The model under review builds one solid part; all positions refer to its coordinate system, in mm. Face numbers are marked on the shaded views. A direction names the side the tool comes from. Coordinates: 2 decimals unless noted, no trailing zeros. Loops run counter-clockwise (first coordinate to the right, second up) from the corner with the lowest first, then second, coordinate; pieces in that order, holes last. Notation, with made-up numbers: (-0.75, 53) - (33.25, 53) arc R29 ccw to (33.25, 73) - close; hole circle Ø11 at (3, 42.25). An arc over 180 degrees is marked (long way). One line per item, written item: value. Start each with the question number.
1. We need section B-B, the plane y = 53.5. Give the boundary of the cut face in (x, z), then the cut area to 3 significant figures.
2. Insertion check: P1, Ø10, axis at x = 12.5, z = 32, coming from the -Y side; P2, Ø12, axis at y = 43.5, z = 45.5, coming from the +X side; P3, Ø8, axis at x = -28.5, z = 54, coming from the +Y side; P4, Ø1, axis at x = 20.5, y = 46.5, coming from the -Z side. Each pin has a flat end and moves straight along its axis. Give the tip position at first contact, or say it passes through.
3. We need section C-C, the plane x = -35.5. Give the boundary of the cut face in (y, z), then the cut area to 3 significant figures.
4. For the marked faces 1 and 2, list the 3-axis set-ups (+Z, -Z, +X, -X, +Y, -Y) from which the entire face can be reached by the end or side of a thin tool; tool diameter is ignored.
5. We need section D-D, the plane x = 0. Give the boundary of the cut face in (y, z), then the cut area to 3 significant figures.
6. To check wall thickness, follow line 1 (X direction, y = 53.75, z = 0); line 2 (Y direction, x = 17, z = 51.5); line 3 (Z direction, x = 9.5, y = 48). State the ranges of each line that lie inside material, in increasing order.
7. We need section A-A, the plane z = 0. Give the boundary of the cut face in (x, y), then the cut area to 3 significant figures.
from build123d import *

# Parameters (mm, degrees)
SKETCH1_R           = 72
BOSS_EXTRUDE4_DEPTH = 50
SKETCH5_R           = 72
SKETCH5_R_2         = 69
BOSS_EXTRUDE5_DEPTH = 7


with BuildPart() as part:
    # Sketch1 → Boss-Extrude4 (new body)
    with BuildSketch(Plane(origin=(0, 0, 0), x_dir=(1, 0, 0), z_dir=(0, 1, 0))):
        with Locations(Location((0, 0, 0), (0, 0, 270))):
            Circle(SKETCH1_R)
    extrude(amount=BOSS_EXTRUDE4_DEPTH)

    # Sketch4 → Cut-Revolve2 (revolve, cut)
    with BuildSketch(Plane.XY, mode=Mode.PRIVATE) as cut_revolve2_sk:
        with BuildLine():
            Line((0, 50), (42, 50))
            ThreePointArc((42, 50), (29.69848481, 20.30151519), (0, 8))
            Line((0, 8), (0, 50))
        make_face()
    revolve(cut_revolve2_sk.sketch.rotate(Axis((0, 50, 0), (0, -1, 0)), 180), axis=Axis((0, 50, 0), (0, -1, 0)), mode=Mode.SUBTRACT)

    # Sketch5 → Boss-Extrude5 (add)
    with BuildSketch(Plane(origin=(0, 50, 0), x_dir=(1, 0, 0), z_dir=(0, 1, 0))):
        with Locations(Location((0, 0, 0), (0, 0, 270))):
            Circle(SKETCH5_R)
        with Locations(Location((0, 0, 0), (0, 0, 270))):
            Circle(SKETCH5_R_2, mode=Mode.SUBTRACT)
    extrude(amount=BOSS_EXTRUDE5_DEPTH)


solid = part.part
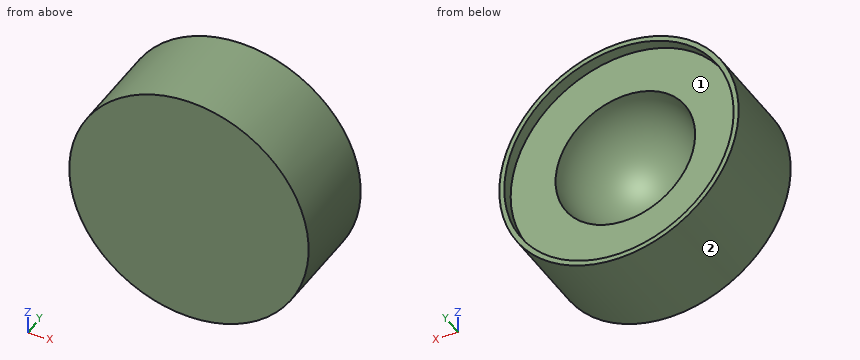
Findings below:
1. outline: circle Ø144 at (0, 0); hole circle Ø138 at (0, 0)
1. area: 1,330 mm2
2. P1: y = 0
2. P2: x = 60.2
2. P3: y = 50
2. P4: z = -69.17
3. outline: (0, -62.64) - (57, -62.64) - (57, -59.17) - (50, -59.17) - (50, -22.44) arc R22.44 cw to (50, 22.44) - (50, 59.17) - (57, 59.17) - (57, 62.64) - (0, 62.64) - close
3. area: 5,520 mm2
4. face 1: +Y
4. face 2: +Y, -Y
5. outline: (0, -72) - (57, -72) - (57, -69) - (50, -69) - (50, -42) arc R42 cw to (50, 42) - (50, 69) - (57, 69) - (57, 72) - (0, 72) - close
5. area: 4,470 mm2
6. line 1: -72 to -69, 69 to 72
6. line 2: 0 to 50
6. line 3: -71.37 to -40.86, 40.86 to 71.37
7. outline: (-72, 0) - (72, 0) - (72, 57) - (69, 57) - (69, 50) - (42, 50) arc R42 cw to (-42, 50) - (-69, 50) - (-69, 57) - (-72, 57) - close
7. area: 4,470 mm2
